```python
from build123d import *

# Parameters (mm, degrees)
F0_W     = 100
F0_H     = 40
F1_DEPTH = 30
F2_DEPTH = 5
F0_W_2   = 21
F0_H_2   = 6
F3_DEPTH = 13
F0_H_3   = 2
F4_DEPTH = 25
F5_R     = 5


with BuildPart() as f1:
    # F0 (on Top) → F1 (new body)
    with BuildSketch(Plane.XY):
        Polygon((0, 60), (0, 0), (120, 0), (120, 60), (112, 60), (112, 58), (112, 52), (91, 52), (91, 58), (91, 60), (49, 60), (49, 58), (49, 52), (28, 52), (28, 58), (28, 60), align=None)
        with Locations((60, 30)):
            Rectangle(F0_W, F0_H, mode=Mode.SUBTRACT)
    extrude(amount=F1_DEPTH)

    # F0 (on Top) → F2 (join)
    with BuildSketch(Plane.XY):
        with Locations((60, 30)):
            Rectangle(F0_W, F0_H)
    extrude(amount=F2_DEPTH)

    # F0 (on Top) → F3 (join)
    with BuildSketch(Plane.XY):
        with Locations((38.5, 55)):
            Rectangle(F0_W_2, F0_H_2)
        with Locations((101.5, 55)):
            Rectangle(F0_W_2, F0_H_2)
    extrude(amount=F3_DEPTH)

    # F0 (on Top) → F4 (join)
    with BuildSketch(Plane.XY):
        with Locations((38.5, 59)):
            Rectangle(F0_W_2, F0_H_3)
        with Locations((101.5, 59)):
            Rectangle(F0_W_2, F0_H_3)
    extrude(amount=F4_DEPTH)

    # F5
    f5_edges = [f1.edges().sort_by_distance(p)[0] for p in [
        (0, 0, 15),
        (120, 0, 15),
        (120, 60, 15),
        (0, 60, 15),
    ]]
    fillet(f5_edges, radius=F5_R)


solid = f1.part
```
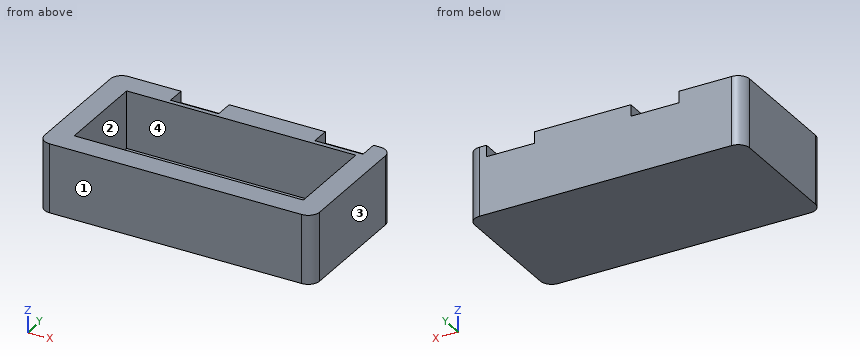
Source: CAD feature listing. Evaluate the final solid. Frame: model axes, mm. Face numbers are marked on the shaded views. Coordinates: 2 decimals unless noted, no trailing zeros. Loops run counter-clockwise (first coordinate to the right, second up) from the corner with the lowest first, then second, coordinate; pieces in that order, holes last. Notation, with made-up numbers: M -5,50.5 L 17,50.5 A18 ccw 17,72.5 Z; hole C 28.5,1 d7. An arc over 180 degrees is marked long. Use a Markdown table: item, result. Add a question column.
Q1. First-contact query: pin 1 (1.6 mm diameter, centred on x = 98, y = 59, fed in from +Z); pin 2 (4 mm diameter, centred on y = 57.5, z = 20.5, fed in from -X); pin 3 (3 mm diameter, centred on x = 43.5, y = 54.5, fed in from +Z). Flat tips, straight axial feed; report the tip coordinate or a pass-through.
Q2. Material intervals for L1, parallel to Y at x = 101, z = 23.75; L2, parallel to X at y = 41, z = 28.25; L3, parallel to Y at x = 54, z = 12, sorted ascending.
Q3. Section query C-C, the plane y = 38. Return loops of the section in (x, z), and give its area (3 significant figures).
Q4. Section query D-D, the plane x = 107. Return loops of the section in (y, z).
Q5. Section query B-B, the plane x = 75. Return loops of the section in (y, z).
Q6. Draft query along Y for the marked faces 1, 2, 3 and 4. Return one class per face: pulls with the +Y half, pulls with the -Y half, needs draft (parallel to the pull), parting line crosses it, or undercut.
Q7. Section query A-A, the plane z = 18.25. Return loops of the section in (x, y), and give its area (3 significant figures).
Result:
| question | item | result |
|---|---|---|
| 1 | pin 1 | stops at z = 25 |
| 1 | pin 2 | stops at x = 0.03 |
| 1 | pin 3 | stops at z = 13 |
| 2 | L1 | y = 0 to 10, 50 to 52, 58 to 60 |
| 2 | L2 | x = 0 to 10, 110 to 120 |
| 2 | L3 | y = 0 to 10, 50 to 60 |
| 3 | outline | M 0,0 L 120,0 L 120,30 L 110,30 L 110,5 L 10,5 L 10,30 L 0,30 Z |
| 3 | area | 1,100 mm2 |
| 4 | outline | M 0,0 L 60,0 L 60,25 L 58,25 L 58,13 L 52,13 L 52,30 L 50,30 L 50,5 L 10,5 L 10,30 L 0,30 Z |
| 5 | outline | M 0,0 L 60,0 L 60,30 L 50,30 L 50,5 L 10,5 L 10,30 L 0,30 Z |
| 6 | face 1 | pulls with the -Y half |
| 6 | face 2 | undercut |
| 6 | face 3 | needs draft |
| 6 | face 4 | undercut |
| 7 | outline | M 0,5 A5 ccw 5,0 L 115,0 A5 ccw 120,5 L 120,55 A5 ccw 115,60 L 5,60 A5 ccw 0,55 Z; hole M 10,10 L 110,10 L 110,50 L 10,50 Z; hole M 28,52 L 49,52 L 49,58 L 28,58 Z; hole M 91,52 L 112,52 L 112,58 L 91,58 Z |
| 7 | area | 2,930 mm2 |
